Work out the finished part from the listing and answer in its coordinate system (mm). A direction names the side the tool comes from. Coordinates: 2 decimals unless noted, no trailing zeros. Loops run counter-clockwise (first coordinate to the right, second up) from the corner with the lowest first, then second, coordinate; pieces in that order, holes last. Notation, with made-up numbers: M 65,86.25 L 117,86.25 A21 cw 117,99.25 Z; hole C 13.5,-31 d11. An arc over 180 degrees is marked long. Write each question's results on one line, items separated by ' | '.
```python
from build123d import *

# Parameters (mm, degrees)
BOSS_EXTRUDE1_DEPTH = 60
FILLET1_R           = 12
FILLET2_R           = 12
CUT_EXTRUDE1_REACH  = 130.561
SKETCH4_R           = 5
CUT_EXTRUDE2_REACH  = 130.561
SKETCH5_R           = 6


with BuildPart() as part:
    # Sketch2 → Boss-Extrude1 (new body)
    with BuildSketch(Plane.XY):
        with BuildLine():
            Line((0, -12), (0, -88))
            Line((0, -88), (-12, -88))
            Line((-12, -88), (-12, 12))
            Line((-12, 12), (0, 12))
            Line((0, 12), (0, 54))
            Line((0, 54), (12, 54))
            Line((12, 54), (12, 30))
            ThreePointArc((12, 30), (13.464466094, 26.464466094), (17, 25))
            Line((17, 25), (49, 25))
            ThreePointArc((49, 25), (52.535533906, 26.464466094), (54, 30))
            Line((54, 30), (54, 54))
            Line((54, 54), (60, 54))
            Line((60, 54), (60, 11))
            Line((60, 11), (48, 11))
            Line((48, 11), (48, 6))
            Line((48, 6), (60, 6))
            Line((60, 6), (60, 0))
            Line((60, 0), (12, 0))
            ThreePointArc((12, 0), (3.514718626, -3.514718626), (0, -12))
        make_face()
    extrude(amount=BOSS_EXTRUDE1_DEPTH)

    # Fillet1
    fillet1_edges = [part.edges().sort_by_distance(p)[0] for p in [
        (0, 12, 30),
    ]]
    fillet(fillet1_edges, radius=FILLET1_R - 0.0001)  # a hair under: the kernel refuses the full size

    # Fillet2
    fillet2_edges = [part.edges().sort_by_distance(p)[0] for p in [
        (6, 54, 0),
        (57, 54, 0),
        (-6, -88, 0),
        (57, 54, 60),
        (-6, -88, 60),
        (6, 54, 60),
    ]]
    fillet(fillet2_edges, radius=FILLET2_R)

    # Sketch4 → Cut-Extrude1 (cut, up to next)
    with BuildSketch(Plane.ZY.offset(12), mode=Mode.PRIVATE) as cut_extrude1_sk1:
        with Locations(Location((15, -68, 0), (0, 0, 270))):
            Circle(SKETCH4_R)
    cut_extrude1_tool1 = extrude(cut_extrude1_sk1.sketch, amount=-CUT_EXTRUDE1_REACH, mode=Mode.PRIVATE) & part.part
    # Sketch4 → Cut-Extrude1 (cut, up to next)
    with BuildSketch(Plane.ZY.offset(12), mode=Mode.PRIVATE) as cut_extrude1_sk2:
        with Locations(Location((45, -68, 0), (0, 0, 270))):
            Circle(SKETCH4_R)
    cut_extrude1_tool2 = extrude(cut_extrude1_sk2.sketch, amount=-CUT_EXTRUDE1_REACH, mode=Mode.PRIVATE) & part.part
    # Sketch4 → Cut-Extrude1 (cut, up to next)
    with BuildSketch(Plane.ZY.offset(12), mode=Mode.PRIVATE) as cut_extrude1_sk3:
        with Locations(Location((15, 39, 0), (0, 0, 270))):
            Circle(SKETCH4_R)
    cut_extrude1_tool3 = extrude(cut_extrude1_sk3.sketch, amount=-CUT_EXTRUDE1_REACH, mode=Mode.PRIVATE) & part.part
    # Sketch4 → Cut-Extrude1 (cut, up to next)
    with BuildSketch(Plane.ZY.offset(12), mode=Mode.PRIVATE) as cut_extrude1_sk4:
        with Locations(Location((45, 39, 0), (0, 0, 270))):
            Circle(SKETCH4_R)
    cut_extrude1_tool4 = extrude(cut_extrude1_sk4.sketch, amount=-CUT_EXTRUDE1_REACH, mode=Mode.PRIVATE) & part.part
    add(cut_extrude1_tool1.solids().sort_by_distance((-12, -68, 15))[0], mode=Mode.SUBTRACT)
    add(cut_extrude1_tool2.solids().sort_by_distance((-12, -68, 45))[0], mode=Mode.SUBTRACT)
    add(cut_extrude1_tool3.solids().sort_by_distance((-12, 39, 15))[0], mode=Mode.SUBTRACT)
    add(cut_extrude1_tool4.solids().sort_by_distance((-12, 39, 45))[0], mode=Mode.SUBTRACT)

    # Sketch5 → Cut-Extrude2 (cut, up to next)
    with BuildSketch(Plane(origin=(60, 0, 0), x_dir=(0, 0, -1), z_dir=(1, 0, 0)), mode=Mode.PRIVATE) as cut_extrude2_sk1:
        with Locations(Location((-30, 42, 0), (0, 0, 90))):
            Circle(SKETCH5_R)
    cut_extrude2_tool1 = extrude(cut_extrude2_sk1.sketch, amount=-CUT_EXTRUDE2_REACH, mode=Mode.PRIVATE) & part.part
    add(cut_extrude2_tool1.solids().sort_by_distance((60, 42, 30))[0], mode=Mode.SUBTRACT)


solid = part.part
```
1) Find section A-A, the plane y = -68. Give the vertices of the cut face in (x, z), and give its area (3 significant figures).
Check result:
outline: M -12,0 L 0,0 L 0,10 L -12,10 Z; M -12,20 L 0,20 L 0,40 L -12,40 Z; M -12,50 L 0,50 L 0,60 L -12,60 Z | area: 480 mm^2
2) For a pull along X with two mould halves and no side action, classify faces 6 (the face through (52, 26, 30)), 7 (the face through (-6.08, -66.92, 10.12)), 8 (the face through (48, 9, 30)) as released by +X, released by -X, zero draft, split by the parting line, or undercut.
Check result:
face 6: undercut | face 7: zero draft | face 8: released by +X
3) Find section D-D, the plane y = 39. Give the vertices of the cut face in (x, z), and give its area (3 significant figures).
Check result:
outline: M 0,0 L 12,0 L 12,10 L 0,10 Z; M 0,20 L 12,20 L 12,40 L 0,40 Z; M 0,50 L 12,50 L 12,60 L 0,60 Z; M 54,0 L 60,0 L 60,24.8 L 54,24.8 Z; M 54,35.2 L 60,35.2 L 60,60 L 54,60 Z | area: 778 mm^2
4) Which of the six approach directions +Z, -Z, +X, -X, +Y, -Y give full straight-line access (tool end or side, diameter ignored) to faces 1 (the face through (13, 27, 30)), 2 (the face through (57.042, 40.699, 24.143)), 3 (the face through (-6.08, -84.39, 3.42)), 4 (the face through (6, 43, 48)), 5 (the face through (54, 6, 30))?
Check result:
face 1: +Z, -Z, +Y | face 2: +X | face 3: -Z, +X, -X, -Y | face 4: -X | face 5: +Z, -Z, +X
5) Given pin 1 Ø9.5 at (x, z) = (53, 19.5) entering from -Y; pin 2 Ø15.5 at (y, z) = (42, 30) entering from -X; pin 3 Ø6 at (x, y) = (31, -2) entering from +Z; pin 4 Ø2.5 at (y, z) = (9.5, 16) entering from +X, each flat-ended and moving along its own axis, determine where each tip first touches the part or whether it passes through.
Check result:
pin 1: y = 0 | pin 2: x = 0 | pin 3: z = 60 | pin 4: x = 48
6) Find section C-C, the plane x = 51. Give the vertices of the cut face in (y, z).
Check result:
outline: M 0,0 L 6,0 L 6,60 L 0,60 Z; M 11,0 L 25.42,0 L 25.42,60 L 11,60 Z
7) Find section B-B, the plane z = 45. Give the number of separate pieces and of enclosed holes in the cut face, and give its area (3 significant figures).
Check result:
separate pieces: 3 | enclosed holes: 0 | area: 2,990 mm^2
8) Straight lines are drawn through the part: probe 1 along Z at (x, y) = (-5, -68); probe 2 along X at (y, z) = (-81.5, 27); probe 3 along X at (y, z) = (47, 50). For each, find the intervals that lie inside material, in ascending order. Write a range as [from, to].
Check result:
probe 1: [0, 10], [20, 40], [50, 60] | probe 2: [-12, 0] | probe 3: [0, 12], [54, 60]
